Autodesk Inventor part; units mm, degrees
ref_plane "Work Plane2" through (0, 0, 2.5) normal (0, 0, 1) x (1, 0, 0)
ref_plane "Work Plane8" through (0, 0, 0) normal (0.9238795, 0.3826834, 0) x (0, 0, 1)
ref_plane "Work Plane9" through (0, 0, 0) normal (1, 0, 0) x (0, 1, 0)
sketch "Sketch1" plane through (0, 0, 0) normal (0, 0, 1) x (1, 0, 0)
  circle A0 centre (0, 0) radius 7.5
  dimension "d0" = 15
extrude "Extrusion1" add sketch "Sketch1" along normal blind 5
ref_plane "Work Plane2" through (0, 0, 2.5) normal (0, 0, 1) x (1, 0, 0)
sketch "Sketch2" plane through (0, 0, 0) normal (0, 0, -1) x (-1, 0, 0)
  circle A0 centre (0, 0) radius 7.5
  circle A1 centre (0, 0) radius 6
  dimension "d3" = 12
surface extrude "Pitch Diameter" sketch "Sketch2" against normal through all shown no curves A1
ref_plane "Work Plane8" through (0, 0, 0) normal (0.9238795, 0.3826834, 0) x (0, 0, 1)
ref_plane "Work Plane9" through (0, 0, 0) normal (1, 0, 0) x (0, 1, 0)
spur gear teeth "Spur Gear" teeth 8 pitch diameter 12 tip diameter 15 root diameter 8.25 face width 5 start plane through (0, 0, 0) normal (0, 0, -1) x (-1, 0, 0)
sketch "Sketch3" plane through (0, 0, 5) normal (0, 0, 1) x (1, 0, 0)
  circle A0 centre (0, 0) radius 2.5
  dimension "d49" = 5
extrude "Extrusion2" cut sketch "Sketch3" against normal up to surface (5 mm away)
equation "\"d0\" = da_da"
equation "\"d1\" = da_b"
equation "\"d3\" = da_d"
equation "\"d16\" = da_aw"
equation "\"d43\" = da_aw"
equation "\"d46\" = da_aw"
properties part number "Spur Gear1" material "Steel"
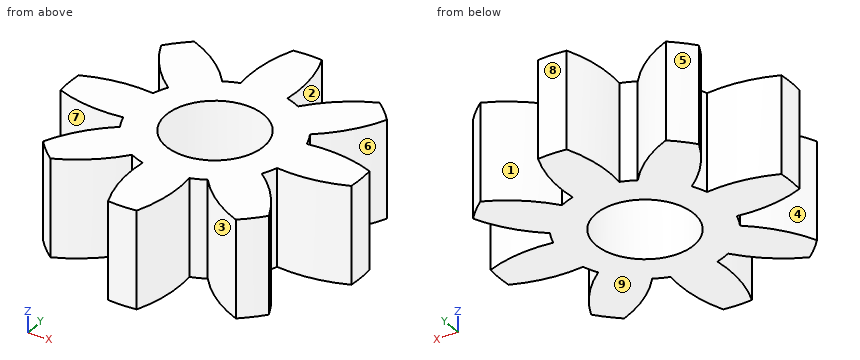
Source: CAD feature listing. Evaluate the final solid. Frame: model axes, mm. Face numbers are marked on the shaded views. A direction names the side the tool comes from. Give positions to 0.01 mm unless a question says otherwise; leave off trailing zeros. Write each loop counter-clockwise with the first axis right and the second up, starting at its lowest first coordinate (ties: lowest second). Pieces come first, ordered by that corner, then holes. Notation, with made-up numbers: (10.25, 9.25) -> (18.25, 9.25) arc R21 ccw to (18.25, 30.25) -> close; hole circle Ø10 at (51.25, 22). An arc over 180 degrees is marked (long way). Write item = value, one per line.
Q1. Mould query, pull axis X, two halves, no side actions, for the marked faces 6, 7, 8 and 9. Classes: +X half, -X half, draft (parallel to the pull), parting line (faces both ways), or undercut.
Here are the results:
face_6 = +X half
face_7 = undercut
face_8 = parting line
face_9 = draft
Q2. Line query: line 1 (Y direction, x = 0, z = 2.1); line 2 (Y direction, x = 5.5, z = 4.05); line 3 (Y direction, x = 5.75, z = 2.6). Output: solid intervals per line, ascending. Write a range as from..to.
Here are the results:
line_1 = -7.5..-2.5, 2.5..7.5
line_2 = -5.1..-4.14, -1.22..1.22, 4.14..5.1
line_3 = -4.82..-4.65, -1.19..1.19, 4.65..4.82
Q3. Cut plane A-A on x = 0. Return loops of the section in (y, z), then the cut area to 3 significant figures.
Here are the results:
outline = (-7.5, 0) -> (-2.5, 0) -> (-2.5, 5) -> (-7.5, 5) -> close; (2.5, 0) -> (7.5, 0) -> (7.5, 5) -> (2.5, 5) -> close
area = 50.0 mm²
Q4. Cut plane D-D on y = -5.5. Return loops of the section in (x, z).
Here are the results:
outline = (-5.1, 0) -> (-4.14, 0) -> (-4.14, 5) -> (-5.1, 5) -> close; (-1.22, 0) -> (1.22, 0) -> (1.22, 5) -> (-1.22, 5) -> close; (4.14, 0) -> (5.1, 0) -> (5.1, 5) -> (4.14, 5) -> close
Q5. First-contact query: pin 1 (3 mm diameter, centred on x = -5.5, z = 3, fed in from -Y); pin 2 (3 mm diameter, centred on y = -1.5, z = 3, fed in from +X); pin 3 (3 mm diameter, centred on y = -4, z = 0.5, fed in from -X). Flat tips, straight axial feed; report the tip coordinate or a pass-through.
Here are the results:
pin_1 = -5.8
pin_2 = 7.5
pin_3 = -5.8
Q6. Reachability of the marked faces 1, 2, 3, 4 and 5 from +Z, -Z, +X, -X, +Y, -Y: full face, straight path, thin tool, end or side. Return the list, or none.
Here are the results:
face_1 = +Z, -Z, +Y
face_2 = +Z, -Z
face_3 = +Z, -Z, -Y
face_4 = +Z, -Z, -X
face_5 = +Z, -Z, -X, +Y
